Can you work these out from the model? Positions are in its coordinate system, mm. Give positions to 0.01 mm unless a question says otherwise; leave off trailing zeros. Loops run counter-clockwise (first coordinate to the right, second up) from the corner with the lowest first, then second, coordinate; pieces in that order, holes last. Notation, with made-up numbers: (63, -37) - (70, -37) arc R15 ccw to (70, -17) - close; hole circle Ø10 at (-16, -32). An arc over 180 degrees is marked (long way). Answer as a JSON object with one key per item and string values. Group by question number.
Item 1: Suppose I cut it at C-C on z = 13.5. Count the separate pieces of the cut face and the enclosed holes in it, and give its area (3 significant figures).
Item 2: Will this pin go through, and if not, where does the flat tip stop? pin 1 (4 mm diameter, centred on x = 9, y = -15.5, fed in from +Z).
Item 3: Suppose I cut it at B-B on x = 8. Write out the boundary of the cut face in (y, z).
Item 4: Suppose I cut it at A-A on y = 2.5. Write out the boundary of the cut face in (x, z), and give its area (3 significant figures).
Item 5: Thinking about a two-plate mould opening in Y: for faces 1 (the flat face through (50, -1, 12)), 2 (the flat face through (-1, -50, 12)), 3 (the flat face through (-1, 50, 12)), which applies, pulls with the +Y half, pulls with the -Y half, needs draft (parallel to the pull), parting line crosses it, or undercut?
Item 6: Please list where these lines run through material, in increasing order: L1, parallel to Y at x = 15.5, z = 22; L2, parallel to Y at x = -5, z = 22.75; L3, parallel to Z at x = -12.5, y = -6.
from build123d import *

# Parameters (mm, degrees)
F0_W     = 100
F0_H     = 100
F1_DEPTH = 25
F2_R     = 0.45
F3_DEPTH = 25.001


with BuildPart() as f1:
    # F0 (on Top) → F1 (new body)
    with BuildSketch(Plane.XY):
        Rectangle(F0_W, F0_H)
    extrude(amount=F1_DEPTH)

    # F2 (on face) → F3 (cut, through all)
    with BuildSketch(Plane.XY.offset(25)):
        with Locations((-49, -49)):
            Circle(F2_R)
        with Locations((-49, -48)):
            Circle(F2_R)
        with Locations((-49, -47)):
            Circle(F2_R)
        with Locations((-49, -46)):
            Circle(F2_R)
        with Locations((-49, -45)):
            Circle(F2_R)
        with Locations((-49, -44)):
            Circle(F2_R)
        with Locations((-49, -43)):
            Circle(F2_R)
        with Locations((-49, -42)):
            Circle(F2_R)
        with Locations((-49, -41)):
            Circle(F2_R)
        with Locations((-48, -49)):
            Circle(F2_R)
        with Locations((-48, -48)):
            Circle(F2_R)
        with Locations((-48, -47)):
            Circle(F2_R)
        with Locations((-48, -46)):
            Circle(F2_R)
        with Locations((-48, -45)):
            Circle(F2_R)
        with Locations((-48, -44)):
            Circle(F2_R)
        with Locations((-48, -43)):
            Circle(F2_R)
        with Locations((-48, -42)):
            Circle(F2_R)
        with Locations((-48, -41)):
            Circle(F2_R)
        with Locations((-47, -49)):
            Circle(F2_R)
        with Locations((-47, -48)):
            Circle(F2_R)
        with Locations((-47, -47)):
            Circle(F2_R)
        with Locations((-47, -46)):
            Circle(F2_R)
        with Locations((-47, -45)):
            Circle(F2_R)
        with Locations((-47, -44)):
            Circle(F2_R)
        with Locations((-47, -43)):
            Circle(F2_R)
        with Locations((-47, -42)):
            Circle(F2_R)
        with Locations((-47, -41)):
            Circle(F2_R)
        with Locations((-46, -49)):
            Circle(F2_R)
        with Locations((-46, -48)):
            Circle(F2_R)
        with Locations((-46, -47)):
            Circle(F2_R)
        with Locations((-46, -46)):
            Circle(F2_R)
        with Locations((-46, -45)):
            Circle(F2_R)
        with Locations((-46, -44)):
            Circle(F2_R)
        with Locations((-46, -43)):
            Circle(F2_R)
        with Locations((-46, -42)):
            Circle(F2_R)
        with Locations((-46, -41)):
            Circle(F2_R)
        with Locations((-45, -49)):
            Circle(F2_R)
        with Locations((-45, -48)):
            Circle(F2_R)
        with Locations((-45, -47)):
            Circle(F2_R)
        with Locations((-45, -46)):
            Circle(F2_R)
        with Locations((-45, -45)):
            Circle(F2_R)
        with Locations((-45, -44)):
            Circle(F2_R)
        with Locations((-45, -43)):
            Circle(F2_R)
        with Locations((-45, -42)):
            Circle(F2_R)
        with Locations((-45, -41)):
            Circle(F2_R)
        with Locations((-44, -49)):
            Circle(F2_R)
        with Locations((-44, -48)):
            Circle(F2_R)
        with Locations((-44, -47)):
            Circle(F2_R)
        with Locations((-44, -46)):
            Circle(F2_R)
        with Locations((-44, -45)):
            Circle(F2_R)
        with Locations((-44, -44)):
            Circle(F2_R)
        with Locations((-44, -43)):
            Circle(F2_R)
        with Locations((-44, -42)):
            Circle(F2_R)
        with Locations((-44, -41)):
            Circle(F2_R)
        with Locations((-43, -49)):
            Circle(F2_R)
        with Locations((-43, -48)):
            Circle(F2_R)
        with Locations((-43, -47)):
            Circle(F2_R)
        with Locations((-43, -46)):
            Circle(F2_R)
        with Locations((-43, -45)):
            Circle(F2_R)
        with Locations((-43, -44)):
            Circle(F2_R)
        with Locations((-43, -43)):
            Circle(F2_R)
        with Locations((-43, -42)):
            Circle(F2_R)
        with Locations((-43, -41)):
            Circle(F2_R)
        with Locations((-42, -49)):
            Circle(F2_R)
        with Locations((-42, -48)):
            Circle(F2_R)
        with Locations((-42, -47)):
            Circle(F2_R)
        with Locations((-42, -46)):
            Circle(F2_R)
        with Locations((-42, -45)):
            Circle(F2_R)
        with Locations((-42, -44)):
            Circle(F2_R)
        with Locations((-42, -43)):
            Circle(F2_R)
        with Locations((-42, -42)):
            Circle(F2_R)
        with Locations((-42, -41)):
            Circle(F2_R)
        with Locations((-41, -49)):
            Circle(F2_R)
        with Locations((-41, -48)):
            Circle(F2_R)
        with Locations((-41, -47)):
            Circle(F2_R)
        with Locations((-41, -46)):
            Circle(F2_R)
        with Locations((-41, -45)):
            Circle(F2_R)
        with Locations((-41, -44)):
            Circle(F2_R)
        with Locations((-41, -43)):
            Circle(F2_R)
        with Locations((-41, -42)):
            Circle(F2_R)
        with Locations((-41, -41)):
            Circle(F2_R)
    extrude(amount=-F3_DEPTH, mode=Mode.SUBTRACT)

    # F5 (on offset) → F6 (revolve, cut)
    with BuildSketch(Plane.XZ):
        with BuildLine():
            Line((0, 10), (0, 25))
            Line((0, 25), (-45, 25))
            ThreePointArc((-45, 25), (-23.7170824513, 13.8487526462), (0, 10))
        make_face()
    revolve(axis=Axis((0, 0, 55), (0, 0, 1)), mode=Mode.SUBTRACT)


solid = f1.part
Worked out:
{
 "1": {"separate pieces": "1", "enclosed holes": "82", "area": "8,340 mm2"},
 "2": {"pin 1": "stops at z = 12.69"},
 "3": {"outline": "(-50, 0) - (50, 0) - (50, 25) - (44.28, 25) arc R74.57 cw to (-44.28, 25) - (-50, 25) - close"},
 "4": {"outline": "(-50, 0) - (50, 0) - (50, 25) - (44.93, 25) arc R74.96 cw to (-44.93, 25) - (-50, 25) - close", "area": "1,580 mm2"},
 "5": {"face 1": "needs draft", "face 2": "pulls with the -Y half", "face 3": "pulls with the +Y half"},
 "6": {"L1": "y = -50 to -37.63, 37.63 to 50", "L2": "y = -50 to -41.53, 41.53 to 50", "L3": "z = 0 to 11.29"}
}
